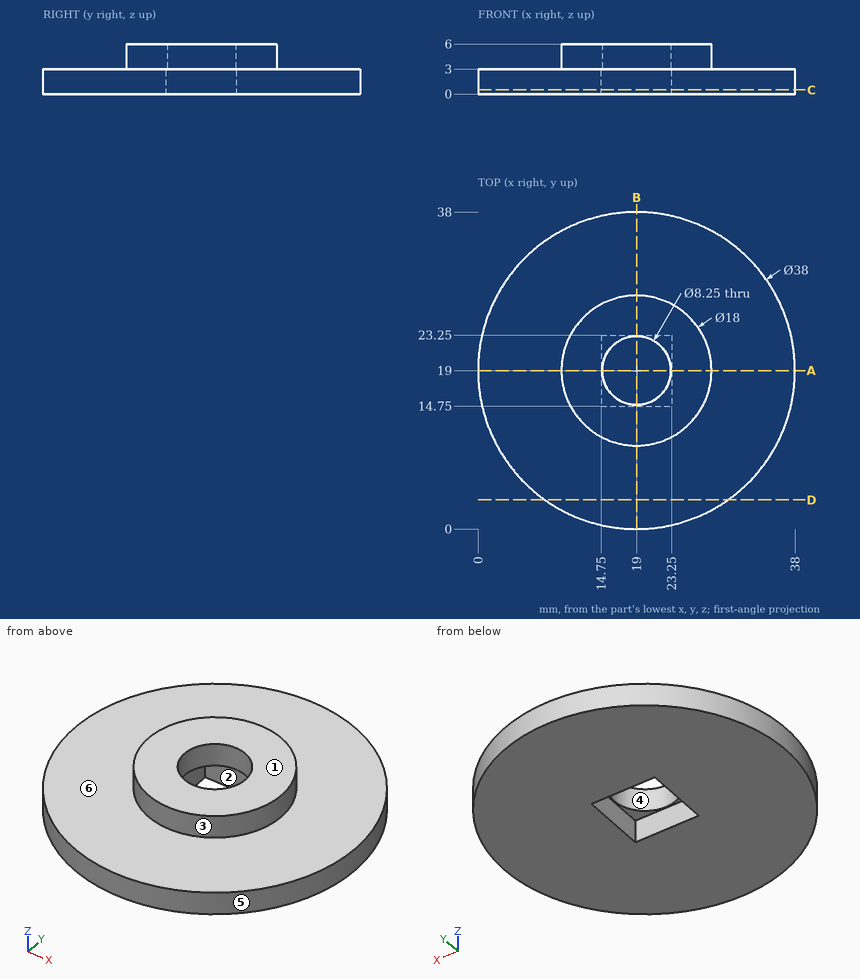
Check sheet for the drawn part. Datum: minimum x, y, z corner. Units: mm. A direction names the side the tool comes from. Coordinates: 2 decimals unless noted, no trailing zeros. Write each loop counter-clockwise with the first axis right and the second up, starting at its lowest first coordinate (ties: lowest second). Pieces come first, ordered by that corner, then holes. Notation, with made-up numbers: M -25.75,21 L -6.75,21 A24 cw -6.75,47 Z; hole C -26,47 d7. An arc over 180 degrees is marked long. One line per item, written item: value.
Item 1: Section check A-A, the plane y = 19. Record the boundary of the cut face in (x, z) (3 decimals), plus the area to 3 significant figures.
Check sheet entries:
outline: M 0,0 L 14.75,0 L 14.75,3 L 14.875,3 L 14.875,6 L 10,6 L 10,3 L 0,3 Z; M 23.125,3 L 23.25,3 L 23.25,0 L 38,0 L 38,3 L 28,3 L 28,6 L 23.125,6 Z
area: 118 mm^2
Item 2: Section check D-D, the plane y = 3.5. Record the boundary of the cut face in (x, z).
Check sheet entries:
outline: M 8.01,0 L 29.99,0 L 29.99,3 L 8.01,3 Z
Item 3: Gauge pin test, flat ends, axial feed: pin 1 Ø6.5 at (x, y) = (19, 19) entering from -Z; pin 2 Ø1.5 at (x, z) = (19, 1.5) entering from +Y; pin 3 Ø2 at (y, z) = (10.5, 1.5) entering from -X; pin 4 Ø2 at (x, z) = (7, 2.5) entering from -Y. Record the tip position at first contact, or that the pin passes through.
Check sheet entries:
pin 1: passes through
pin 2: stops at y = 38
pin 3: stops at x = 1.54
pin 4: stops at y = 3.51
Item 4: Section check C-C, the plane z = 0.5. Record the boundary of the cut face in (x, y), plus the area to 3 significant figures.
Check sheet entries:
outline: C 19,19 d38; hole M 14.75,14.75 L 23.25,14.75 L 23.25,23.25 L 14.75,23.25 Z
area: 1,060 mm^2
Item 5: Mould release check, pull along Y, two halves, no side actions. Record for the marked faces 4, 5 and 6: pulls with the +Y half, pulls with the -Y half, needs draft (parallel to the pull), parting line crosses it, or undercut.
Check sheet entries:
face 4: undercut
face 5: parting line crosses it
face 6: needs draft
Item 6: Access from +Z, -Z, +X, -X, +Y, -Y to the whole of each face (thin tool, end or side, straight path). Record for the marked faces 1, 2 and 3.
Check sheet entries:
face 1: +Z, +X, -X, +Y, -Y
face 2: -Z
face 3: +Z
Item 7: Scan lines: line 1 along Y through (x, z) = (19, 3.8) (3 decimals); line 2 along Z through (x, y) = (28, 8); line 3 along X through (y, z) = (20.5, 0.55). Record each from-to range of solid material in increasing order.
Check sheet entries:
line 1: y = 10 to 14.875, 23.125 to 28
line 2: z = 0 to 3
line 3: x = 0.06 to 14.75, 23.25 to 37.94
